from build123d import *

# Parameters (mm, degrees)
BOX001_W        = 10
BOX001_H        = 50
BOX001_DEPTH    = 3
FILLET001_R     = 2
BOX_W           = 10
BOX_H           = 50
BOX_DEPTH       = 3
BOX_PITCH_ANGLE = -60
FILLET_R        = 2


with BuildPart() as fillet001:
    # Box001 → Box001 (new body)
    with BuildSketch(Plane(origin=(20, -60, -60.5), x_dir=(1, 0, 0), z_dir=(0, 0, 1))):
        with Locations((5, 25)):
            Rectangle(BOX001_W, BOX001_H)
    extrude(amount=BOX001_DEPTH)

    # Fillet001
    fillet001_edges = [fillet001.edges().sort_by_distance(p)[0] for p in [
        (30, -35, -60.5),
    ]]
    fillet(fillet001_edges, radius=FILLET001_R)


with BuildPart() as obj1:
    # Box → Box (new body)
    with BuildSketch(Plane.XY):
        with Locations((5, 25)):
            Rectangle(BOX_W, BOX_H)
    extrude(amount=BOX_DEPTH)


with BuildPart() as obj1_1:
    # Box pitch: moved
    add(obj1.part.rotate(Axis((0, 0, 0), (0, 1, 0)), BOX_PITCH_ANGLE))


with BuildPart() as obj1_2:
    # Box placement: moved
    add(obj1_1.part.moved(Location((30, -60, -60.5))))

    # Fillet
    fillet_edges = [obj1_2.edges().sort_by_distance(p)[0] for p in [
        (30, -35, -60.5),
        (35, -35, -51.839746),
    ]]
    fillet(fillet_edges, radius=FILLET_R)


with BuildPart() as obj1_3:
    # Fillet placement: moved
    add(obj1_2.part.moved(Location((-0.5, 0, -0.5))))

    # Fusion: union Fillet001
    add(fillet001.part)


solid = obj1_3.part
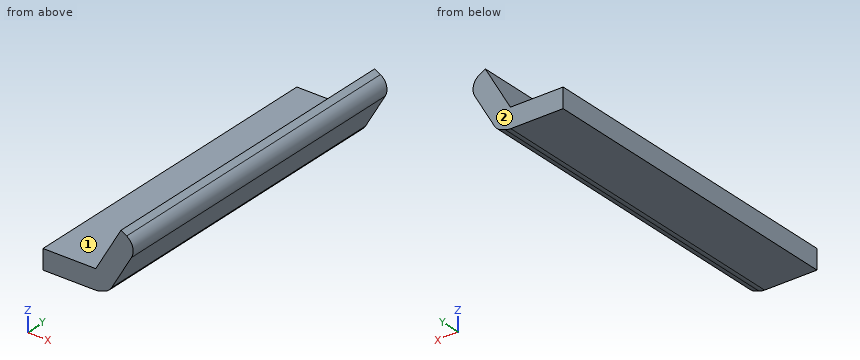
Geometry: final body of the model. Coordinates: model frame, mm. Face numbers are marked on the shaded views. A direction names the side the tool comes from. Round coordinates to 2 decimals unless told otherwise and drop trailing zeros. Loops run counter-clockwise (first coordinate to the right, second up) from the corner with the lowest first, then second, coordinate; pieces in that order, holes last. Notation, with made-up numbers: (-33, 45.25) - (7, 45.25) arc R18 cw to (7, 52.25) - close; hole circle Ø8 at (-29, -24.5). An arc over 180 degrees is marked (long way). Write each question's results on one line, items separated by ' | '. Start each with the question number.
1) Access query for the marked faces 1 and 2. Directions: +Z, -Z, +X, -X, +Y, -Y. A direction counts if a zero-diameter tool reaches every point of the face in a straight line with its end or side. Return the directions, or none.
2) First-contact query: P1, Ø4, axis at y = -22, z = -54, coming from the -X side; P2, Ø2.5, axis at x = 25.5, y = -40.5, coming from the +Z side; P3, Ø1, axis at y = -45.5, z = -56, coming from the +X side. Flat tips, straight axial feed; report the tip coordinate or a pass-through.
3) Cut plane B-B on x = 26.75. Return loops of the section in (y, z).
4) Line query: probe 1 along X at (y, z) = (-24.5, -53.25); probe 2 along Z at (x, y) = (26.5, -44); probe 3 along X at (y, z) = (-18, -59.25). Output: solid intervals per line, ascending. Write a range as [from, to].
5) Cut plane A-A on y = -35. Return loops of the section in (x, z).
6) Cut plane C-C on z = -52.5. Return loops of the section in (x, y), then the cut area to 3 significant figures.
Verdict:
1) face 1: +Z, -X, +Y, -Y | face 2: +Z, -Z, +X, -X, +Y
2) P1: stops at x = 28.92 | P2: stops at z = -57.5 | P3: stops at x = 32.68
3) outline: (-60, -60.5) - (-10, -60.5) - (-10, -57.5) - (-60, -57.5) - close
4) probe 1: x = [30.51, 33.76] | probe 2: z = [-60.5, -57.5] | probe 3: x = [20, 30.51]
5) outline: (20, -60.5) - (28, -60.5) arc R2 ccw to (28.95, -60.26) arc R2 ccw to (30.5, -59.27) - (33.5, -54.07) arc R2 ccw to (32.77, -51.34) - (31.9, -50.84) - (28.06, -57.5) - (20, -57.5) - close
6) outline: (30.94, -60) - (33.68, -60) - (33.68, -10) - (30.94, -10) - close | area: 137 mm2
